Source: CAD feature listing. Evaluate the final solid. Frame: model axes, mm. A direction names the side the tool comes from. Round coordinates to 2 decimals unless told otherwise and drop trailing zeros. Write each loop counter-clockwise with the first axis right and the second up, starting at its lowest first coordinate (ties: lowest second). Pieces come first, ordered by that corner, then holes.
from build123d import *

# Parameters (mm, degrees)
SKETCH1_R           = 5
BOSS_EXTRUDE1_DEPTH = 2
SKETCH2_R           = 1.4
BOSS_EXTRUDE2_DEPTH = 4.3
BOSS_EXTRUDE3_DEPTH = 2.2
SKETCH4_R           = 1.1
BOSS_EXTRUDE4_DEPTH = 4.8
BOSS_EXTRUDE7_DEPTH = 2.2
SKETCH8_R           = 1
BOSS_EXTRUDE8_DEPTH = 2
CUT_EXTRUDE1_REACH  = 24.425
SKETCH9_R           = 1
CIRPATTERN1_COUNT   = 8
SKETCH10_R          = 2
CUT_EXTRUDE3_DEPTH  = 1
FILLET6_R           = 0.5


with BuildPart() as part:
    # Sketch1 → Boss-Extrude1 (new body)
    with BuildSketch(Plane.XY):
        Circle(SKETCH1_R)
    extrude(amount=-BOSS_EXTRUDE1_DEPTH)

    # Sketch2 → Boss-Extrude2 (add)
    with BuildSketch(Plane.XY):
        with Locations(Location((0, 0, 0), (0, 0, 180))):
            Circle(SKETCH2_R)
    extrude(amount=BOSS_EXTRUDE2_DEPTH)

    # Sketch3 → Boss-Extrude3 (add)
    with BuildSketch(Plane.XY.offset(4.3)):
        with BuildLine():
            Line((0, -2.5), (-10.6, -2.5))
            ThreePointArc((-10.6, -2.5), (-13.1, 0), (-10.6, 2.5))
            Line((-10.6, 2.5), (0, 2.5))
            ThreePointArc((0, 2.5), (2.5, 0), (0, -2.5))
        make_face()
    extrude(amount=BOSS_EXTRUDE3_DEPTH)

    # Sketch4 → Boss-Extrude4 (add)
    with BuildSketch(Plane.XY.offset(6.5)):
        with Locations((-10.6, 0)):
            Circle(SKETCH4_R)
    extrude(amount=BOSS_EXTRUDE4_DEPTH)

    # Sketch7 → Boss-Extrude7 (add)
    with BuildSketch(Plane.XY.offset(11.3)):
        with BuildLine():
            Line((-10.6, 2.5), (0, 2.5))
            ThreePointArc((0, 2.5), (2.5, 0), (0, -2.5))
            Line((0, -2.5), (-10.6, -2.5))
            ThreePointArc((-10.6, -2.5), (-13.1, 0), (-10.6, 2.5))
        make_face()
    extrude(amount=BOSS_EXTRUDE7_DEPTH)

    # Sketch8 → Boss-Extrude8 (add)
    with BuildSketch(Plane.XY.offset(13.5)):
        Circle(SKETCH8_R)
    extrude(amount=BOSS_EXTRUDE8_DEPTH)

    # Sketch9 → Cut-Extrude1 (cut, up to next)
    with BuildSketch(Plane(origin=(0, 0, -2), x_dir=(-1, 0, 0), z_dir=(0, 0, -1)), mode=Mode.PRIVATE) as cut_extrude1_sk1:
        with Locations((5, 0)):
            Circle(SKETCH9_R)
    cut_extrude1_tool1 = extrude(cut_extrude1_sk1.sketch, amount=-CUT_EXTRUDE1_REACH, mode=Mode.PRIVATE) & part.part
    cut_extrude1 = cut_extrude1_tool1.solids().sort_by_distance((-5, 0, -2))[0]
    add(cut_extrude1, mode=Mode.SUBTRACT)

    # CirPattern1: Cut-Extrude1 ×8 about axis
    cirpattern1_axis = Axis((0, 0, 0), (0, 0, 1))
    for i in range(1, CIRPATTERN1_COUNT):
        add(cut_extrude1.rotate(cirpattern1_axis, i * 360 / CIRPATTERN1_COUNT), mode=Mode.SUBTRACT)

    # Sketch10 → Cut-Extrude3 (cut)
    with BuildSketch(Plane(origin=(0, 0, -2), x_dir=(-1, 0, 0), z_dir=(0, 0, -1))):
        Circle(SKETCH10_R)
    extrude(amount=-CUT_EXTRUDE3_DEPTH, mode=Mode.SUBTRACT)

    # Fillet6
    fillet6_edges = [part.edges().sort_by_distance(p)[0] for p in [
        (2, 0, -1),
        (2, 0, -2),
    ]]
    fillet(fillet6_edges, radius=FILLET6_R - 0.0001)  # a hair under: the kernel refuses the full size


solid = part.part
1) Section query C-C on x = -1.75. State how many separate pieces and enclosed holes the cut face has, then the cut area to 3 significant figures.
Taken from the geometry:
separate pieces: 3
enclosed holes: 0
area: 38.9 mm2
2) Section query D-D on z = 7.5. Return the cut outline in (x, y), then the cut area to 3 significant figures.
Taken from the geometry:
outline: circle Ø2.2 at (-10.6, 0)
area: 3.80 mm2
3) Section query B-B on y = 4.5. Return the cut outline in (x, z), then the cut area to 3 significant figures.
Taken from the geometry:
outline: (-2.18, -2) - (-0.87, -2) - (-0.87, 0) - (-2.18, 0) - close; (0.87, -2) - (2.18, -2) - (2.18, 0) - (0.87, 0) - close
area: 5.25 mm2
4) Material intervals for line 1 (Z direction, x = -4, y = 0.5); line 2 (Z direction, x = -1.5, y = -0.25); line 3 (Z direction, x = -4.5, y = 0.75), sorted ascending.
Taken from the geometry:
line 1: z = -2 to 0, 4.3 to 6.5, 11.3 to 13.5
line 2: z = -1 to 0, 4.3 to 6.5, 11.3 to 13.5
line 3: z = 4.3 to 6.5, 11.3 to 13.5
5) Contact query for flat-ended pins moving along their axis: P1, Ø5, axis at y = 3, z = 0.5, coming from the -X side; P2, Ø4, axis at x = -7, y = 1, coming from the -Z side; P3, Ø2.5, axis at x = -3, z = 6, coming from the +Y side. Output: stop coordinate, or through.
Taken from the geometry:
P1: stops at x = -4.9
P2: stops at z = 4.3
P3: stops at y = 2.5
6) Pull-direction query (Z, two-part tool) for faces 6 (the face through (-5, 0, 13.5)), 7 (the face through (4.614, -1.926, -0.986)), 8 (the face through (-2, 2, -2)), 9 (the face through (-10.01, 0.93, 8.87)); classes: released by +Z, released by -Z, zero draft, split by the parting line, or undercut.
Taken from the geometry:
face 6: released by +Z
face 7: zero draft
face 8: released by -Z
face 9: undercut
7) Reachability of faces 1 (the face through (4.625, 1.901, -0.986)), 2 (the face through (2.5, 0.1, 12.4)), 3 (the face through (1, 1.2, 0)), 4 (the face through (-5, -2.5, 5)), 5 (the face through (-5, 2.5, 12)) from +Z, -Z, +X, -X, +Y, -Y: full face, straight path, thin tool, end or side. Return the list, or none.
Taken from the geometry:
face 1: +Z, -Z, +X, +Y
face 2: +Z, +X
face 3: none
face 4: +Z, +X, -X, -Y
face 5: +Z, +X, -X, +Y
